from build123d import *

# Parameters (mm, degrees)
F1_DEPTH = 457.2
F2_R     = 6.35
F3_DEPTH = 50.801


with BuildPart() as f1:
    # F0 (on Front) → F1 (new body)
    with BuildSketch(Plane.XZ):
        with BuildLine():
            ThreePointArc((25.4, 22.225), (24.470064, 24.470064), (22.225, 25.4))
            Line((22.225, 25.4), (-22.225, 25.4))
            ThreePointArc((-22.225, 25.4), (-24.470064, 24.470064), (-25.4, 22.225))
            Line((-25.4, 22.225), (-25.4, -22.225))
            ThreePointArc((-25.4, -22.225), (-24.470064, -24.470064), (-22.225, -25.4))
            Line((-22.225, -25.4), (22.225, -25.4))
            ThreePointArc((22.225, -25.4), (24.470064, -24.470064), (25.4, -22.225))
            Line((25.4, -22.225), (25.4, 22.225))
        make_face()
        with BuildLine():
            Line((-17.4625, 20.6375), (17.4625, 20.6375))
            ThreePointArc((17.4625, 20.6375), (19.707564, 19.707564), (20.6375, 17.4625))
            Line((20.6375, 17.4625), (20.6375, -17.4625))
            ThreePointArc((20.6375, -17.4625), (19.707564, -19.707564), (17.4625, -20.6375))
            Line((17.4625, -20.6375), (-17.4625, -20.6375))
            ThreePointArc((-17.4625, -20.6375), (-19.707564, -19.707564), (-20.6375, -17.4625))
            Line((-20.6375, -17.4625), (-20.6375, 17.4625))
            ThreePointArc((-20.6375, 17.4625), (-19.707564, 19.707564), (-17.4625, 20.6375))
        make_face(mode=Mode.SUBTRACT)
    extrude(amount=F1_DEPTH)

    # F2 (on face) → F3 (cut, through all)
    with BuildSketch(Plane.YZ.offset(25.4)):
        with Locations((-431.8, 0)):
            Circle(F2_R)
        with Locations((-25.4, 0)):
            Circle(F2_R)
    extrude(amount=-F3_DEPTH, mode=Mode.SUBTRACT)


solid = f1.part
Geometry check sheet. Reference: the model listing, model coordinates, mm. A direction names the side the tool comes from. Give positions to 0.01 mm unless a question says otherwise; leave off trailing zeros. Loops run counter-clockwise (first coordinate to the right, second up) from the corner with the lowest first, then second, coordinate; pieces in that order, holes last. Notation, with made-up numbers: M 30,54.5 L 59,54.5 A29 ccw 59,93.5 Z; hole C -10,-39.75 d4. An arc over 180 degrees is marked long. Answer as a JSON object with one key per item and string values. Group by question number.
Item 1: Sectioned sample at D-D on x = -10.5. Record the boundary of the cut face in (y, z), plus the area to 3 significant figures.
Item 2: Material ranges on L1, parallel to X at y = -144.5, z = -18; L2, parallel to Z at x = -15, y = -223.5; L3, parallel to Z at x = 21.9, y = -431.8, recorded low to high.
Item 3: Gauge pin test, flat end, axial feed: pin 1 (11.5 mm diameter, centred on y = -431.8, z = 0, fed in from +X). Record the tip position at first contact, or that the pin passes through.
Item 4: Access from +Z, -Z, +X, -X, +Y, -Y to the whole of each face (thin tool, end or side, straight path). Record for faces 4 (the flat face through (0, -225, -20.638)), 5 (the flat face through (22, 0, 0)).
Item 5: Mould release check, pull along X, two halves, no side actions. Record for faces 1 (the flat face through (25.4, -225, 0)), 2 (the flat face through (0, -225, -25.4)), 3 (the flat face through (-20.638, -225, 0)): pulls with the +X half, pulls with the -X half, needs draft (parallel to the pull), parting line crosses it, or undercut.
Item 6: Sectioned sample at B-B on z = 0. Record the boundary of the cut face in (x, y), plus the area to 3 significant figures.
Findings below:
{
 "1": {"outline": "M -457.2,-25.4 L 0,-25.4 L 0,-20.64 L -457.2,-20.64 Z; M -457.2,20.64 L 0,20.64 L 0,25.4 L -457.2,25.4 Z", "area": "4,350 mm2"},
 "2": {"L1": "-25.4 to -20.59, 20.59 to 25.4", "L2": "-25.4 to -20.64, 20.64 to 25.4", "L3": "-25.4 to -6.35, 6.35 to 25.4"},
 "3": {"pin 1": "through"},
 "4": {"face 4": "+Y, -Y", "face 5": "+Z, -Z, +X, -X, +Y"},
 "5": {"face 1": "pulls with the +X half", "face 2": "needs draft", "face 3": "undercut"},
 "6": {"outline": "M -25.4,-457.2 L -20.64,-457.2 L -20.64,-438.15 L -25.4,-438.15 Z; M -25.4,-425.45 L -20.64,-425.45 L -20.64,-31.75 L -25.4,-31.75 Z; M -25.4,-19.05 L -20.64,-19.05 L -20.64,0 L -25.4,0 Z; M 20.64,-457.2 L 25.4,-457.2 L 25.4,-438.15 L 20.64,-438.15 Z; M 20.64,-425.45 L 25.4,-425.45 L 25.4,-31.75 L 20.64,-31.75 Z; M 20.64,-19.05 L 25.4,-19.05 L 25.4,0 L 20.64,0 Z", "area": "4,110 mm2"}
}
